For this review, take the finished solid that the model builds, in its own axes (mm). A direction names the side the tool comes from. Coordinates: 2 decimals unless noted, no trailing zeros. Write each loop counter-clockwise with the first axis right and the second up, starting at its lowest first coordinate (ties: lowest second). Pieces come first, ordered by that corner, then holes.
```python
from build123d import *

# Parameters (mm, degrees)
BOSS_EXTRUDE1_DEPTH      = 20
BOSS_EXTRUDE1_DEPTH_BACK = 20
FILLET4_R                = 7.5
FILLET5_R                = 7.5
FILLET6_R                = 7.5
FILLET7_R                = 7.5
CUT_EXTRUDE6_DEPTH       = 137.106575888


with BuildPart() as part:
    # Sketch1 → Boss-Extrude1 (new, two sides: drawn at the far end of the back side and taken through both)
    with BuildSketch(Plane.XY.offset(-BOSS_EXTRUDE1_DEPTH_BACK)):
        with BuildLine():
            Line((125, 0), (-125, 0))
            Line((-125, 0), (-125, 14))
            ThreePointArc((-125, 14), (-77.640903187, 39.335842187), (-25, 50))
            Line((-25, 50), (25, 50))
            ThreePointArc((25, 50), (77.640903187, 39.335842187), (125, 14))
            Line((125, 14), (125, 0))
        make_face()
    extrude(amount=BOSS_EXTRUDE1_DEPTH + BOSS_EXTRUDE1_DEPTH_BACK)

    # Fillet4
    fillet4_edges = [part.edges().sort_by_distance(p)[0] for p in [
        (-125, 14, 0),
    ]]
    fillet(fillet4_edges, radius=FILLET4_R)

    # Fillet5
    fillet5_edges = [part.edges().sort_by_distance(p)[0] for p in [
        (125, 14, 0),
    ]]
    fillet(fillet5_edges, radius=FILLET5_R)

    # Fillet6
    fillet6_edges = [part.edges().sort_by_distance(p)[0] for p in [
        (125, 0, 0),
    ]]
    fillet(fillet6_edges, radius=FILLET6_R)

    # Fillet7
    fillet7_edges = [part.edges().sort_by_distance(p)[0] for p in [
        (-125, 0, 0),
    ]]
    fillet(fillet7_edges, radius=FILLET7_R)

    # Sketch3 → Cut-Extrude6 (cut, through all)
    with BuildSketch(Plane(origin=(0, 0, 0), x_dir=(1, 0, 0), z_dir=(0, 1, 0))):
        with BuildLine():
            ThreePointArc((-59.997253933, 9), (-40.06, 0), (-59.997253933, -9))
            Line((-59.997253933, -9), (-125, -9))
            Line((-125, -9), (-125, 9))
            Line((-125, 9), (-59.997253933, 9))
        make_face()
        with BuildLine():
            Line((125, 9), (59.997253933, 9))
            ThreePointArc((59.997253933, 9), (40.06, 0), (59.997253933, -9))
            Line((59.997253933, -9), (125, -9))
            Line((125, -9), (125, 9))
        make_face()
    extrude(amount=CUT_EXTRUDE6_DEPTH, mode=Mode.SUBTRACT)


solid = part.part
```
Q1. Add section D-D (x = 52.06). State the section outline as (y, z) points.
Ans:
outline: (0, -20) - (46.52, -20) - (46.52, -12) - (0, -12) - close; (0, 12) - (46.52, 12) - (46.52, 20) - (0, 20) - close
Q2. Clearance check with flat-ended pins moving along their axes: pin 1 Ø12 at (x, z) = (-85, 11.5) entering from +Y; pin 2 Ø13.5 at (x, y) = (101.5, 30) entering from -Z; pin 3 Ø12 at (y, z) = (24, 8) entering from -X. State where each tip first meets the part, or that it passes through.
Ans:
pin 1: stops at y = 38.84
pin 2: stops at z = -20
pin 3: stops at x = -119.25
Q3. Draft analysis for pull direction Z (two halves, no side actions). For faces 1 (the cylindrical face through (124.184, 13.572, 14.577)), 2 (the flat face through (-86, 17, -9)), 3 (the flat face through (2, 20, -20)), state which applies: +Z half, -Z half, draft (parallel to the pull), parting line (faces both ways), or undercut.
Ans:
face 1: draft
face 2: undercut
face 3: -Z half
Q4. Add section C-C (y = 42). State the section outline as (x, z) points.
Ans:
outline: (-69.68, -20) - (69.68, -20) - (69.68, -9) - (60, -9) arc R12 cw (long way) to (60, 9) - (69.68, 9) - (69.68, 20) - (-69.68, 20) - (-69.68, 9) - (-60, 9) arc R12 cw (long way) to (-60, -9) - (-69.68, -9) - close
Q5. Add section B-B (z = 15). State the section outline as (x, y) points.
Ans:
outline: (-125, 7.5) arc R7.5 ccw to (-117.5, 0) - (117.5, 0) arc R7.5 ccw to (125, 7.5) - (125, 10.17) arc R7.5 ccw to (121.83, 16.29) arc R185 ccw to (25, 50) - (-25, 50) arc R185 ccw to (-121.83, 16.29) arc R7.5 ccw to (-125, 10.17) - close
Q6. Tool access review of faces 4 (the flat face through (85, 17, 9)), 5 (the flat face through (-85, 17, 9)), 6 (the cylindrical face through (-122.745, 2.139, -14.423)): name each direction out of +Z, -Z, +X, -X, +Y, -Y from which nothing blocks a thin tool from reaching the whole face with its end or side.
Ans:
face 4: +X, +Y, -Y
face 5: -X, +Y, -Y
face 6: +Z, -Z, -X, -Y
Q7. Add section A-A (x = 87). State the section outline as (y, z) points.
Ans:
outline: (0, -20) - (35.68, -20) - (35.68, -9) - (0, -9) - close; (0, 9) - (35.68, 9) - (35.68, 20) - (0, 20) - close
Q8. For probe 1 along Z at (x, y) = (111.5, 14.5); probe 2 along X at (y, z) = (11, 0); probe 3 along X at (y, z) = (6.5, 16), list the stretches that pass through material, from the lowest coordinate up.
Ans:
probe 1: z = -20 to -9, 9 to 20
probe 2: x = -40.06 to 40.06
probe 3: x = -124.93 to 124.93
